Source: CAD feature listing. Evaluate the final solid. Frame: model axes, mm. Face numbers are marked on the shaded views. A direction names the side the tool comes from. Give positions to 0.01 mm unless a question says otherwise; leave off trailing zeros. Loops run counter-clockwise (first coordinate to the right, second up) from the corner with the lowest first, then second, coordinate; pieces in that order, holes last.
from build123d import *

# Parameters (mm, degrees)
SKETCH1_R           = 17.5
BOSS_EXTRUDE1_DEPTH = 5
FILLET1_R           = 3
SKETCH2_R           = 2.5
BOSS_EXTRUDE2_DEPTH = 10


with BuildPart() as part:
    # Sketch1 → Boss-Extrude1 (new, symmetric)
    with BuildSketch(Plane.XY):
        Circle(SKETCH1_R)
    extrude(amount=BOSS_EXTRUDE1_DEPTH, both=True)

    # Fillet1
    fillet1_edges = [part.edges().sort_by_distance(p)[0] for p in [
        (-17.5, 0, -5),
        (-17.5, 0, 5),
    ]]
    fillet(fillet1_edges, radius=FILLET1_R)

    # Sketch2 → Boss-Extrude2 (add, symmetric)
    with BuildSketch(Plane.XY):
        Circle(SKETCH2_R)
    extrude(amount=BOSS_EXTRUDE2_DEPTH, both=True)


solid = part.part
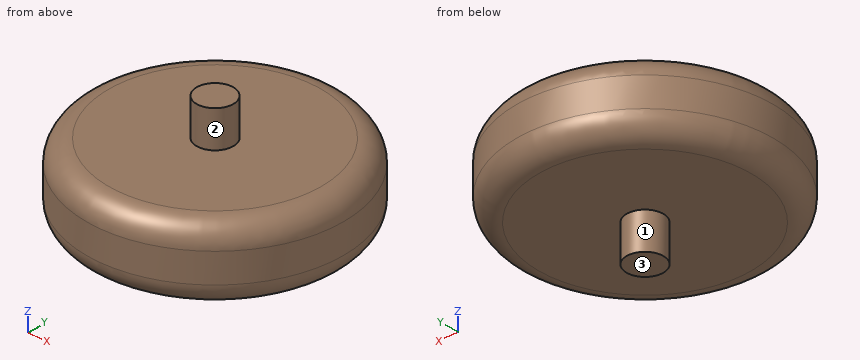
1) Contact query for flat-ended pins moving along their axis: P1, Ø8.5, axis at x = -1.5, y = -5.5, coming from the +Z side; P2, Ø1, axis at x = -2.5, y = 2.5, coming from the -Z side; P3, Ø12, axis at y = -10.5, z = -6.5, coming from the +X side; P4, Ø5, axis at y = -13.5, z = -5.5, coming from the +X side. Output: stop coordinate, or through.
Checks:
P1: stops at z = 10
P2: stops at z = -5
P3: stops at x = 16.4
P4: stops at x = 12.23
2) Ray query, probe 1 along Z at (x, y) = (0.5, -8); probe 2 along Y at (x, z) = (-1.5, -1.25); probe 3 along Y at (x, z) = (8.5, -3.5). Return the intervals inside material, ascending.
Checks:
probe 1: z = -5 to 5
probe 2: y = -17.44 to 17.44
probe 3: y = -14.84 to 14.84
3) Reachability of the marked faces 1, 2 and 3 from +Z, -Z, +X, -X, +Y, -Y: full face, straight path, thin tool, end or side. Return the list, or none.
Checks:
face 1: -Z
face 2: +Z
face 3: -Z, +X, -X, +Y, -Y
4) Cut plane A-A (x = 0). Return loops of the section in (y, z).
Checks:
outline: (-17.5, -2) arc R3 ccw to (-14.5, -5) - (-2.5, -5) - (-2.5, -10) - (2.5, -10) - (2.5, -5) - (14.5, -5) arc R3 ccw to (17.5, -2) - (17.5, 2) arc R3 ccw to (14.5, 5) - (2.5, 5) - (2.5, 10) - (-2.5, 10) - (-2.5, 5) - (-14.5, 5) arc R3 ccw to (-17.5, 2) - close
5) Cut plane D-D (z = -0.75). Return loops of the section in (x, y), and give its area (3 significant figures).
Checks:
outline: circle Ø35 at (0, 0)
area: 962 mm2
6) Cut plane C-C (z = -6.75). Return loops of the section in (x, y).
Checks:
outline: circle Ø5 at (0, 0)
